Job drawing, mm, ordinate dimensions from the low corner. One solid piece. A direction names the side the tool comes from. Give positions to 0.01 mm unless a question says otherwise; leave off trailing zeros. Write each loop counter-clockwise with the first axis right and the second up, starting at its lowest first coordinate (ties: lowest second). Pieces come first, ordered by that corner, then holes. Notation, with made-up numbers: (-23, 31.25) -> (34, 31.25) arc R27 ccw to (34, 65.25) -> close; hole circle Ø1 at (-0.75, 51). An arc over 180 degrees is marked (long way). Put each result on its own line as item: value. Start each with the question number.
Item 1: Tool access for the marked faces 1, 2 and 3: list every direction of +Z, -Z, +X, -X, +Y, -Y with a clear straight run to the whole face (end or side of a thin tool).
Item 2: Flat gauge pins, fed straight in: pin 1 Ø2.5 at (x, y) = (50.5, 70) entering from +Z; pin 2 Ø3 at (y, z) = (59, 23) entering from +X; pin 3 Ø1.5 at (x, y) = (55, 34.5) entering from +Z. Where does each tip first touch, or does it go through?
Item 3: Drill centre lines: line 1 along X through (y, z) = (70, 26.95); line 2 along Z through (x, y) = (40, 2.4); line 3 along Y through (x, z) = (25, 27). Where is each one in solid material? Low to high.
Item 4: Slice it at C-C, the plane x = 60.5. List the corners of the cut face in (y, z).
Item 5: Slice it at B-B, the plane y = 70. List the corners of the cut face in (x, z), plus the area to 3 significant figures.
Item 6: Slice it at D-D, the plane x = 20. List the corners of the cut face in (y, z).
Item 7: Slice it at A-A, the plane z = 40. List the corners of the cut face in (x, y).
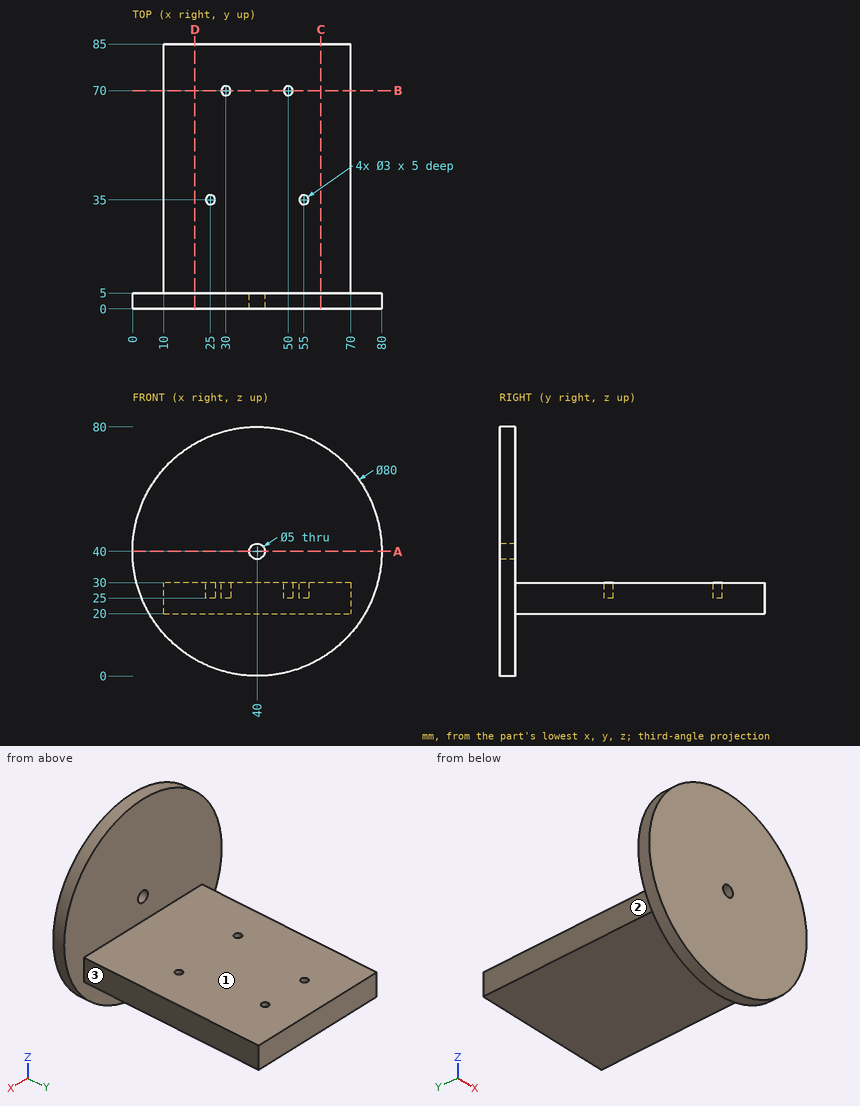
Values follow:
1. face 1: +Z, +X, -X, +Y
1. face 2: +Z, -Z, -X, +Y
1. face 3: +Z, -Z, +X, +Y
2. pin 1: z = 30
2. pin 2: x = 70
2. pin 3: z = 25
3. line 1: 10 to 28.5, 31.5 to 48.5, 51.5 to 70
3. line 2: 0 to 37.5, 42.5 to 80
3. line 3: 0 to 33.5, 36.5 to 85
4. outline: (0, 5.65) -> (5, 5.65) -> (5, 20) -> (85, 20) -> (85, 30) -> (5, 30) -> (5, 74.35) -> (0, 74.35) -> close
5. outline: (10, 20) -> (70, 20) -> (70, 30) -> (51.5, 30) -> (51.5, 25) -> (48.5, 25) -> (48.5, 30) -> (31.5, 30) -> (31.5, 25) -> (28.5, 25) -> (28.5, 30) -> (10, 30) -> close
5. area: 570 mm2
6. outline: (0, 5.36) -> (5, 5.36) -> (5, 20) -> (85, 20) -> (85, 30) -> (5, 30) -> (5, 74.64) -> (0, 74.64) -> close
7. outline: (0, 0) -> (37.5, 0) -> (37.5, 5) -> (0, 5) -> close; (42.5, 0) -> (80, 0) -> (80, 5) -> (42.5, 5) -> close
